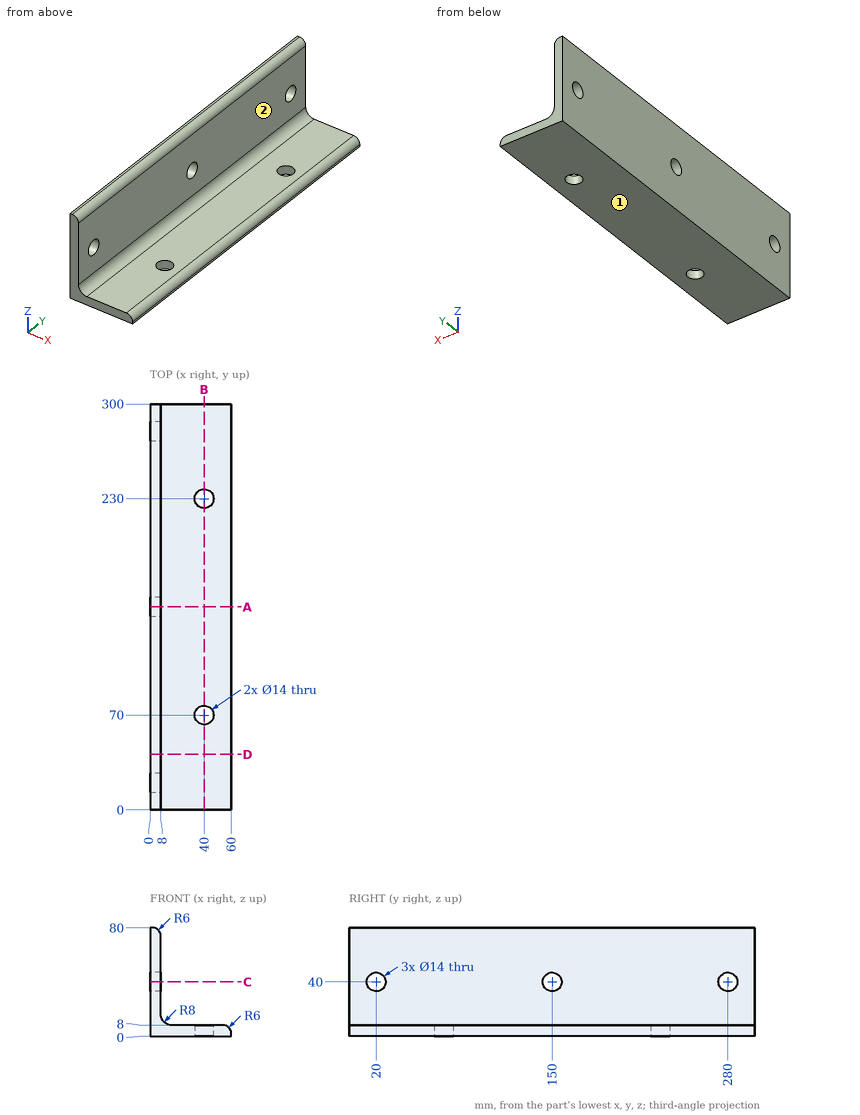
Print and shaded views of the part. All mm, measured from the part's lowest x, y and z. A direction names the side the tool comes from. Coordinates: 2 decimals unless noted, no trailing zeros. Order: outer loops, then holes, each group sorted by start corner. A loop starts at its lowest first (then second) coordinate and runs counter-clockwise, first axis right, second up.
(1) Slice it at C-C, the plane z = 40. Write the cut outline in (x, y).
Check sheet entries:
outline: (0, 0) - (8, 0) - (8, 13) - (0, 13) - close; (0, 27) - (8, 27) - (8, 143) - (0, 143) - close; (0, 157) - (8, 157) - (8, 273) - (0, 273) - close; (0, 287) - (8, 287) - (8, 300) - (0, 300) - close
(2) Pin check, flat tips, straight feed: pin 1 Ø3 at (y, z) = (111.5, 23) entering from +X; pin 2 Ø18 at (x, y) = (40, 230) entering from +Z. Stop position of each tip, or through.
Check sheet entries:
pin 1: stops at x = 8
pin 2: stops at z = 8
(3) Slice it at B-B, the plane x = 40. Write the cut outline in (y, z), and give its area (3 significant figures).
Check sheet entries:
outline: (0, 0) - (63, 0) - (63, 8) - (0, 8) - close; (77, 0) - (223, 0) - (223, 8) - (77, 8) - close; (237, 0) - (300, 0) - (300, 8) - (237, 8) - close
area: 2,180 mm2
(4) Probe L1, parallel to Y at x = 40, z = 5.75; L2, parallel to X at y = 230, z = 2; L3, parallel to Z at x = 49.5, y = 98. List the from-to ranges inside material, lowest first.
Check sheet entries:
L1: y = 0 to 63, 77 to 223, 237 to 300
L2: x = 0 to 33, 47 to 60
L3: z = 0 to 8
(5) Tool access for the marked faces 1 and 2: list every direction of +Z, -Z, +X, -X, +Y, -Y with a clear straight run to the whole face (end or side of a thin tool).
Check sheet entries:
face 1: -Z, +X, -X, +Y, -Y
face 2: +Z, +X, +Y, -Y
(6) Slice it at D-D, the plane y = 41. Write the cut outline in (x, z).
Check sheet entries:
outline: (0, 0) - (60, 0) - (60, 2) arc R6 ccw to (54, 8) - (16, 8) arc R8 cw to (8, 16) - (8, 74) arc R6 ccw to (2, 80) - (0, 80) - close
(7) Slice it at A-A, the plane y = 150. Write the cut outline in (x, z).
Check sheet entries:
outline: (0, 0) - (60, 0) - (60, 2) arc R6 ccw to (54, 8) - (16, 8) arc R8 cw to (8, 16) - (8, 33) - (0, 33) - close; (0, 47) - (8, 47) - (8, 74) arc R6 ccw to (2, 80) - (0, 80) - close
